Part model, mm, in its own coordinate system. Face numbers are marked on the shaded views. Round coordinates to 2 decimals unless told otherwise and drop trailing zeros. Write each loop counter-clockwise with the first axis right and the second up, starting at its lowest first coordinate (ties: lowest second). Pieces come first, ordered by that corner, then holes. Notation, with made-up numbers: M 61.5,21.5 L 98.5,21.5 A31 cw 98.5,50.5 Z; hole C 73,80 d7. An arc over 180 degrees is marked long. Use a Markdown table: item, result. Add a question column.
1) Wall check: probe 1 along Y at (x, z) = (0, 2.15); probe 2 along Z at (x, y) = (22, -2); probe 3 along Y at (x, z) = (22, 1.65). Give the ranges that are in metal, low to high.
2) Slice it at C-C on y = 0. Give the number of separate pieces and of enclosed holes in the cut face, plus the area to 3 significant figures.
3) Slice it at A-A on x = 9.5. Write the cut outline in (y, z).
4) Slice it at B-B on z = -32.5. Write the cut outline in (x, y), plus the area to 3 significant figures.
5) Two-plate mould, pull along Z, no slides. Class the marked faces 1, 2 and 3: released by +Z, released by -Z, zero draft, split by the parting line, or undercut.
6) Drop flat-ended pins along their axis: P1, Ø3.5, axis at x = 11, z = 2, coming from the -Y side; P2, Ø11, axis at x = 14.5, y = -1.5, coming from the -Z side; P3, Ø1.5, axis at x = 36, z = -6.5, coming from the -Y side. Give the stop position or say it passes through.
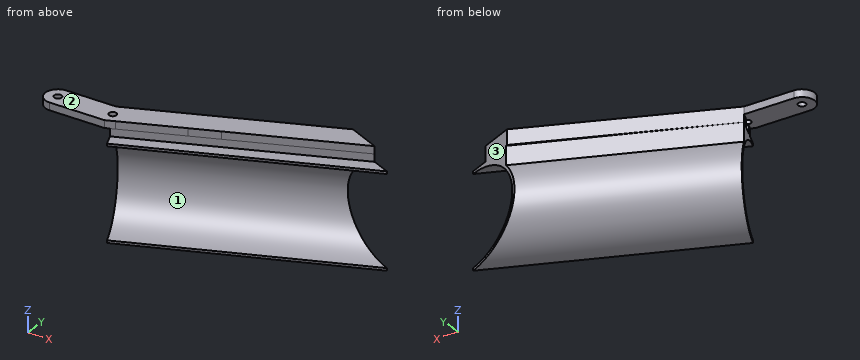
```python
from build123d import *

# Parameters (mm, degrees)
SKETCH1_R           = 1.5
BOSS_EXTRUDE1_DEPTH = 3
EXTRUDE_1_DEPTH     = 3
EXTRUDE_2_DEPTH     = 3
EXTRUDE_3_REACH     = 100.745
CUT_EXTRUDE_1_DEPTH = 45


with BuildPart() as part:
    # Sketch1 → Boss-Extrude1 (new body)
    # profile 1 of 2: a face of its own
    with BuildSketch(Plane.XY):
        with BuildLine():
            Line((20.05, 5), (0, 5))
            ThreePointArc((0, 5), (-5, 0), (0, -5))
            Line((0, -5), (22, -5))
            Line((22, -5), (25.516973514, -3.553997369))
            ThreePointArc((25.516973514, -3.553997369), (26.624391141, 1.901317064), (22, 5))
            Line((22, 5), (20.05, 5))
        make_face()
        Circle(SKETCH1_R, mode=Mode.SUBTRACT)
        with Locations((22, 0)):
            Circle(SKETCH1_R, mode=Mode.SUBTRACT)
    # profile 2 of 2: a face of its own
    with BuildSketch(Plane.XY):
        with BuildLine():
            Line((46.409029503, 15.837507263), (20.05, 5))
            Line((20.05, 5), (22, 5))
            ThreePointArc((22, 5), (26.624391141, 1.901317064), (25.516973514, -3.553997369))
            Line((25.516973514, -3.553997369), (48.359029503, 5.837507263))
            Line((48.359029503, 5.837507263), (58.872830999, 10.16025367))
            Line((58.872830999, 10.16025367), (53.359871826, 12.67140304))
            Line((53.359871826, 12.67140304), (46.409029503, 15.837507263))
        make_face()
    extrude(amount=BOSS_EXTRUDE1_DEPTH)

    # 草图1 → 凸台-拉伸1 (add)
    with BuildSketch(Plane.XY.offset(3)):
        Polygon((46.409029503, 15.837507263), (58.872830999, 10.16025367), (111.008388469, 31.59577286), (98.544586973, 37.273026453), align=None)
    extrude(amount=-EXTRUDE_1_DEPTH)

    # 草图4 → 凸台-拉伸2 (add)
    with BuildSketch(Plane(origin=(0, 0, 0), x_dir=(-1, 0, 0), z_dir=(0, 0, -1))):
        with BuildLine():
            Line((-111.008388469, 31.59577286), (-98.544586973, 37.273026453))
            Line((-98.544586973, 37.273026453), (-19.990187018, 4.97540791))
            Line((-19.990187018, 4.97540791), (-21.063636635, 2.318021494))
            ThreePointArc((-21.063636635, 2.318021494), (-24.318021494, 0.936363365), (-22.936363365, -2.318021494))
            Line((-22.936363365, -2.318021494), (-23.732077199, -4.287856967))
            Line((-23.732077199, -4.287856967), (-111.008388469, 31.59577286))
        make_face()
    extrude(amount=EXTRUDE_2_DEPTH)

    # 凸台-拉伸3: up to this plane
    extrude_3_end = Plane(origin=(98.544586973, 37.273026453, -70.058401543), z_dir=(0.4145222599320868, 0.9100391727946636, 0))
    # 草图5 → 凸台-拉伸3 (add, up to the surface)
    with BuildSketch(Plane(origin=(18.913747244, 7.640196631, 0), x_dir=(0.3745453459539944, -0.9272085977945863, 0), z_dir=(-0.9272085977945863, -0.3745453459539944, 0)), mode=Mode.PRIVATE) as extrude_3_sk1:
        with BuildLine():
            Line((17.949999281, -3), (17.949999281, -4))
            ThreePointArc((17.949999281, -4), (-0.050000719, -22), (17.949999281, -40))
            Line((17.949999281, -40), (17.949999281, -41))
            ThreePointArc((17.949999281, -41), (0.910251194, -30.405176091), (2.873990521, -10.43652475))
            Line((2.873990521, -10.43652475), (2.873990521, -3))
            Line((2.873990521, -3), (17.949999281, -3))
        make_face()
    extrude_3_tool1 = split(extrude(extrude_3_sk1.sketch, amount=-EXTRUDE_3_REACH, mode=Mode.PRIVATE), bisect_by=extrude_3_end, keep=Keep.BOTH, mode=Mode.PRIVATE)
    add(extrude_3_tool1.solids().sort_by_distance((20.149314, 4.581481, -6.718262))[0])

    # 草图6 → 切除-拉伸1 (cut, symmetric)
    with BuildSketch(Plane(origin=(0, 0, 0), x_dir=(-1, 0, 0), z_dir=(0, 0, -1))):
        Polygon((-118.12130065, 28.35584592), (-94.278560376, 39.216198833), (-90.467733039, 37.676817461), (-114.310473313, 26.816464549), align=None)
    extrude(amount=CUT_EXTRUDE_1_DEPTH, both=True, mode=Mode.SUBTRACT)


solid = part.part
```
Entries:
| question | item | result |
|---|---|---|
| 1 | probe 1 | y = -5 to -1.5, 1.5 to 5 |
| 1 | probe 2 | z = 0 to 3 |
| 1 | probe 3 | y = -5 to -1.5, 1.5 to 5.8 |
| 2 | separate pieces | 4 |
| 2 | enclosed holes | 0 |
| 2 | area | 205 mm^2 |
| 3 | outline | M -5,0 L 5,0 L 5,3 L -5,3 Z |
| 4 | outline | M 19.71,5.68 L 20.16,4.55 L 95.96,35.17 L 94.44,35.87 Z |
| 4 | area | 98.6 mm^2 |
| 5 | face 1 | undercut |
| 5 | face 2 | released by +Z |
| 5 | face 3 | zero draft |
| 6 | P1 | stops at y = -5 |
| 6 | P2 | stops at z = 0 |
| 6 | P3 | stops at y = 3.51 |
